Geometry: final body of the model. Coordinates: model frame, mm. A direction names the side the tool comes from. Give positions to 0.01 mm unless a question says otherwise; leave off trailing zeros. Loops run counter-clockwise (first coordinate to the right, second up) from the corner with the lowest first, then second, coordinate; pieces in that order, holes last.
1. Material intervals for line 1 along Z through (x, y) = (22.5, -23); line 2 along Z through (x, y) = (56, 37); line 3 along X through (y, z) = (-27, 0), sorted ascending.
2. Access query for faces 5 (the face through (38, 25, -13.991)), 6 (the face through (41.378, 16.125, -1.656)), 7 (the face through (35, -42, 0)). Directions: +Z, -Z, +X, -X, +Y, -Y. A direction counts if a zero-diameter tool reaches every point of the face in a straight line with its end or side. Return the directions, or none.
3. Section D-D, the plane x = 53. Output: boundary loops of the cut face in (y, z).
4. First-contact query: P1, Ø6, axis at y = 34, z = -3, coming from the +X side; P2, Ø6, axis at x = 5.5, z = -11, coming from the -Y side; P3, Ø6.5, axis at y = -42.5, z = 0, coming from the +X side; P4, Ø10, axis at x = 21, y = -48, coming from the -Z side. Flat tips, straight axial feed; report the tip coordinate or a pass-through.
5. Section A-A, the plane z = 6.5. Output: boundary loops of the cut face in (x, y).
6. Section C-C, the plane y = -44. Output: boundary loops of the cut face in (x, z).
7. Section B-B, the plane x = 18.5. Output: boundary loops of the cut face in (y, z), then the cut area to 3 significant figures.
8. Draft query along X for faces 1 (the face through (38, 26, -12.991)), 2 (the face through (29, 11, 10)), 3 (the face through (81.19, 40.07, -13.5)), 4 (the face through (67.307, 35.619, -13.484)). Return one class per face: +X half, -X half, draft (parallel to the pull), parting line (faces both ways), or undercut.
Autodesk Inventor part; units mm, degrees
ref_plane "YZ Plane" through (0, 0, 0) normal (1, 0, 0) x (0, 1, 0)
ref_plane "XY Plane" through (0, 0, 0) normal (0, 0, 1) x (1, 0, 0)
sketch "Sketch1" plane through (0, 0, 0) normal (0, 0, 1) x (1, 0, 0)
  line L0 (1.879385, 0.68404) -> (82.692951, 30.097773)
  line L1 (0, 0) -> (86, 0) construction
  line L2 (83.888296, 32.661198) -> (77.731933, 49.575665)
  line L3 (77.731933, 49.575665) -> (-6.840403, 18.793852)
  line L4 (-6.840403, 18.793852) -> (-0.68404, 1.879385)
  arc A0 (-0.68404, 1.879385) -> (1.879385, 0.68404) centre (1.195345, 2.563426) ccw
  arc A1 (82.692951, 30.097773) -> (83.888296, 32.661198) centre (82.00891, 31.977158) ccw
  point P0 (84.572336, 30.781813)
  dimension "d0" = 90
  dimension "d1" = 20
  dimension "d2" = 20
  dimension "d9" = 2
extrude "Extrusion1" add sketch "Sketch1" along normal blind 10 and the other way blind 13.991
shell "Shell1" thickness 1 removed faces 3 at (49.541154, 39.315061, -5.994) at (81.836175, 38.299354, 2.003) at (24.256972, 23.017853, 10)
fillet "Fillet1" radius 2 2 edges at (-6.3706, 18.9649, 10) (77.7319, 49.5757, -13.491)
sketch "Sketch2" plane through (1.537365, 1.623733, -12.991) normal (0, 0, 1) x (0.9396926, 0.3420201, 0)
  point P0 (-2, -1)
sketch "Sketch3" plane through (1.537365, 1.623733, -12.991) normal (0, 0, 1) x (0.9396926, 0.3420201, 0)
  circle A0 centre (72, 9) radius 1.5
  line L0 (88, 17) -> (88, 1)
  line L1 (86, 0) -> (0, 0)
  point P0 (-2, -1)
  dimension "d10" = 3
  dimension "d11" = 16
  dimension "d12" = 9
extrude "Extrusion2" cut sketch "Sketch3" against normal through all
ref_plane "Work Plane1" through (0, -95, 0) normal (0, 1, 0) x (-1, 0, 0)
sketch "Sketch4" plane through (0, -95, 0) normal (0, 1, 0) x (-1, 0, 0)
  line L0 (-15, -4) -> (-35, -4)
  line L1 (-35, -4) -> (-35, 4)
  line L2 (-35, 4) -> (-15, 4)
  line L3 (-15, 4) -> (-15, -4)
  point P0 (0, 0)
  point P1 (-25, 4)
  point P2 (-25, -4)
  dimension "d16" = 20
  dimension "d17" = 8
  dimension "d18" = 25
  dimension "d19" = 4
extrude "Extrusion3" add sketch "Sketch4" along normal up to surface surface through (1.879385, 0.68404, 0) normal (0.3420201, -0.9396926, 0)
properties part number "shooter base_3DPrint"
Answers below:
1. line 1: z = -4 to 4
1. line 2: z = -13.99 to -12.99
1. line 3: x = 15 to 35
2. face 5: -Z, +X, -X, +Y, -Y
2. face 6: +Z, +Y
2. face 7: +Z, -Z, +X, -Y
3. outline: (19.29, -13.99) - (40.57, -13.99) - (40.57, -12.99) - (20.35, -12.99) - (20.35, 10) - (19.29, 10) - close
4. P1: stops at x = 84.01
4. P2: stops at y = 0.91
4. P3: stops at x = 35
4. P4: stops at z = -4
5. outline: (-6.84, 18.79) - (-0.68, 1.88) arc R2 ccw to (1.88, 0.68) - (82.69, 30.1) arc R2 ccw to (83.89, 32.66) - (82.95, 32.32) arc R1 cw to (82.35, 31.04) - (1.54, 1.62) arc R1 cw to (0.26, 2.22) - (-5.9, 19.14) - close
6. outline: (15, -4) - (35, -4) - (35, 4) - (15, 4) - close
7. outline: (-95, -4) - (6.73, -4) - (6.73, -13.99) - (28.02, -13.99) - (28.02, -12.99) - (7.8, -12.99) - (7.8, 10) - (6.73, 10) - (6.73, 4) - (-95, 4) - close
7. area: 860 mm2
8. face 1: undercut
8. face 2: draft
8. face 3: +X half
8. face 4: undercut
